CAD build for the part. Positions are in the model's coordinates, mm. Face numbers are marked on the shaded views. A direction names the side the tool comes from. Round coordinates to 2 decimals unless told otherwise and drop trailing zeros. Loops run counter-clockwise (first coordinate to the right, second up) from the corner with the lowest first, then second, coordinate; pieces in that order, holes last.
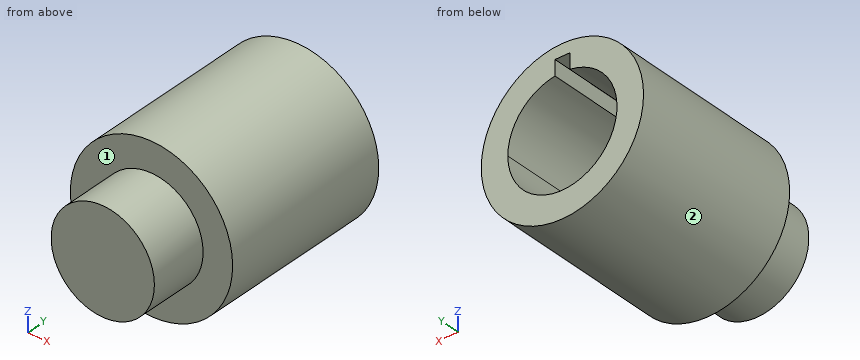
```python
from build123d import *

# Parameters (mm, degrees)
F0_R     = 6.985
F1_DEPTH = 12.7
F2_R     = 6.985
F3_DEPTH = 2.54
F4_R     = 4.445
F5_DEPTH = 5.08


with BuildPart() as f1:
    # F0 (on Front) → F1 (new body)
    with BuildSketch(Plane.XZ):
        Circle(F0_R)
        with BuildLine():
            ThreePointArc((0.635, 4.655897), (3.540089, 3.090043), (4.699, 0))
            ThreePointArc((4.699, 0), (-3.090043, -3.540089), (-0.635, 4.655897))
            Line((-0.635, 4.655897), (-0.635, 5.969))
            Line((-0.635, 5.969), (0, 5.969))
            Line((0, 5.969), (0.635, 5.969))
            Line((0.635, 5.969), (0.635, 4.655897))
        make_face(mode=Mode.SUBTRACT)
    extrude(amount=F1_DEPTH)

    # F2 (on face) → F3 (join)
    with BuildSketch(Plane.XZ.offset(12.7)):
        Circle(F2_R)
    extrude(amount=F3_DEPTH)

    # F4 (on face) → F5 (join)
    with BuildSketch(Plane.XZ.offset(15.24)):
        Circle(F4_R)
    extrude(amount=F5_DEPTH)


solid = f1.part
```
Item 1: Flat gauge pins, fed straight in: P1, Ø1.5, axis at x = -5, y = -4.5, coming from the +Z side; P2, Ø2, axis at x = 2.5, y = -13, coming from the +Z side; P3, Ø1, axis at x = -5.5, y = -5, coming from the +Z side. Where does each tip first touch, or does it go through?
Answers follow:
P1: stops at z = 5.54
P2: stops at z = 6.82
P3: stops at z = 4.88
Item 2: Cut at D-D, the plane y = -17.25. Give the cut face in (x, z) (3 decimals), plus the area to 3 significant figures.
Answers follow:
outline: circle Ø8.89 at (0, 0)
area: 62.1 mm2
Item 3: Cut at C-C, the plane z = 4. Give the cut face in (x, y), plus the area to 3 significant figures.
Answers follow:
outline: (-5.73, -15.24) - (-1.94, -15.24) - (-1.94, -20.32) - (1.94, -20.32) - (1.94, -15.24) - (5.73, -15.24) - (5.73, 0) - (2.47, 0) - (2.47, -12.7) - (-2.47, -12.7) - (-2.47, 0) - (-5.73, 0) - close
area: 132 mm2
Item 4: Cut at B-B, the plane x = 1.5. Give the cut face in (y, z), plus the area to 3 significant figures.
Answers follow:
outline: (-20.32, -4.18) - (-15.24, -4.18) - (-15.24, -6.82) - (0, -6.82) - (0, -4.45) - (-12.7, -4.45) - (-12.7, 4.45) - (0, 4.45) - (0, 6.82) - (-15.24, 6.82) - (-15.24, 4.18) - (-20.32, 4.18) - close
area: 137 mm2
Item 5: Cut at A-A, the plane y = -12.25. Give the cut face in (x, z) (3 decimals), plus the area to 3 significant figures.
Answers follow:
outline: circle Ø13.97 at (0, 0); hole (-0.635, 4.656) arc R4.699 ccw (long way) to (4.699, 0) arc R4.699 ccw to (0.635, 4.656) - (0.635, 5.969) - (-0.635, 5.969) - close
area: 82.3 mm2
Item 6: Probe line 1 (Z direction, x = 0, y = -3.25) (3 decimals); line 2 (Y direction, x = 4.75, z = -3.5); line 3 (X direction, y = -4.25, z = 4.25). List the from-to ranges inside material, lowest first.
Answers follow:
line 1: z = -6.985 to -4.699, 5.969 to 6.985
line 2: y = -15.24 to 0
line 3: x = -5.54 to -2, 2 to 5.54
Item 7: 3-axis set-ups, long thin cutter, end or side, ignore diameter. For the marked faces 1 and 2: which of +Z, -Z, +X, -X, +Y, -Y reach the whole face in a straight line?
Answers follow:
face 1: -Y
face 2: +Y, -Y
